The listing builds one solid part. Answer for the finished solid, in the listing's coordinates (mm). A direction names the side the tool comes from. Round coordinates to 2 decimals unless told otherwise and drop trailing zeros. Loops run counter-clockwise (first coordinate to the right, second up) from the corner with the lowest first, then second, coordinate; pieces in that order, holes last. Notation, with made-up numbers: (31.5, -9) - (49.5, -9) arc R8 ccw to (49.5, -1) - close; hole circle Ø10 at (-32.75, 68). An arc over 180 degrees is marked (long way). One line per item, written item: value.
Autodesk Inventor part; units mm, degrees
ref_plane "YZ Plane" through (0, 0, 0) normal (1, 0, 0) x (0, 1, 0)
ref_plane "XY Plane" through (0, 0, 0) normal (0, 0, 1) x (1, 0, 0)
sketch "Sketch1" plane through (0, 0, 0) normal (0, 1, 0) x (-1, 0, 0)
  circle A0 centre (0, 0) radius 10
  circle A1 centre (0, 0) radius 12.5
  line L0 (12.5, 0) -> (12.5, 50)
  line L1 (-12.5, 0) -> (-12.5, 50)
  line L2 (-12.5, 50) -> (12.5, 50)
  dimension "d0" = 20
  dimension "d1" = 25
  dimension "d2" = 50
extrude "Extrusion1" add sketch "Sketch1" along normal blind 15
sketch "Sketch3" plane through (-12.5, 0, 50) normal (0, 0, 1) x (1, 0, 0)
  point P0 (12.5, 0)
sketch "Sketch4" plane through (-12.5, 0, 50) normal (0, 0, 1) x (1, 0, 0)
  line L0 (25, 0) -> (25, 15)
  line L1 (25, 0) -> (25, 15)
  line L2 (0, 15) -> (25, 15)
  line L3 (25, 15) -> (0, 15)
  line L4 (0, 0) -> (0, 15)
  line L5 (0, 15) -> (0, 0)
  line L6 (0, 0) -> (25, 0)
  line L7 (0, 0) -> (25, 0)
  point P0 (12.5, 0)
extrude "Extrusion3" add sketch "Sketch4" along normal blind 25
sketch "Sketch9" plane through (0, 0, 0) normal (0, -1, 0) x (1, 0, 0)
  line L0 (-12.5, 25) -> (-22.5, 25)
  line L1 (-12.5, 25) -> (12.5, 25)
  line L2 (12.5, 0) -> (12.5, 75)
  line L3 (-12.5, 25) -> (-12.5, 75)
  line L4 (-12.5, 25) -> (-12.5, 75)
  line L5 (-12.5, 75) -> (12.5, 75)
  line L6 (-12.5, 75) -> (12.5, 75)
  line L7 (12.5, 75) -> (12.5, 25)
  line L8 (12.5, 0) -> (12.5, 30)
  line L9 (-12.5, 25) -> (-10.5, 25)
  line L10 (-10.5, 25) -> (-10.5, 75)
  line L11 (-12.5, 75) -> (-12.5, 25)
  line L12 (-10.5, 25) -> (12.5, 30)
  line L13 (-10.5, 25) -> (-10.5, 35)
  line L14 (-10.5, 35) -> (12.5, 35)
  point P0 (0, 0)
  point P1 (12.5, 35)
  dimension "d50" = 30
  dimension "d51" = 2
  dimension "d74" = 10
extrude "Extrusion7" add sketch "Sketch9" along normal blind 13 contours L10 L14 L2 L12
sketch "Sketch10" plane through (0, -13, 0) normal (0, -1, 0) x (1, 0, 0)
  point P0 (0, 0)
ref_plane "Work Plane1" through (0, 7.5, 0) normal (0, 1, 0) x (-1, 0, 0)
mirror "Mirror1" about plane through (0, 7.5, 0) normal (0, 1, 0) of "Extrusion7"
sketch "Sketch15" plane through (-10.5, 15, 25) normal (0.2124296, 0, -0.9771764) x (-0.9771764, 0, -0.2124296)
  line L0 (-23.5372, 0) -> (-23.5372, 13)
  line L1 (-14.7001, 13) -> (-18.6088, 13)
  line L2 (-23.5372, 0) -> (-18.5372, 0)
  line L3 (-18.5372, 0) -> (-18.5372, 13)
  line L4 (-18.5372, 13) -> (-23.5372, 13)
  line L5 (-23.5372, 13) -> (-23.5372, 0)
  line L6 (-23.5372, -28) -> (-24.5994, -28)
  line L7 (-18.6088, -28) -> (-18.6088, 13)
  line L8 (-23.5372, -28) -> (-18.6088, -28)
  line L9 (-18.6088, -28) -> (-18.6088, -15)
  line L10 (-18.6088, -15) -> (-23.5372, -15)
  line L11 (-23.5372, -15) -> (-23.5372, -28)
  point P0 (-4.9496, -15)
  point P1 (-33.0965, -28)
  point P2 (-18.6088, 0)
  point P3 (-23.5372, 13)
  dimension "d66" = 5
extrude "Extrusion9" add sketch "Sketch15" along normal blind 2 contours L0 L4 L7 L2 | L8 L11 L10 L7
sketch "Sketch16" plane through (0, 15, 0) normal (0, 1, 0) x (1, 0, 0)
  circle A0 centre (0, 0) radius 10
  circle A1 centre (0, 0) radius 12.5
  dimension "d69" = 25
extrude "Extrusion10" add sketch "Sketch16" along normal blind 2
sketch "Sketch17" plane through (0, 0, 0) normal (0, -1, 0) x (1, 0, 0)
  circle A0 centre (0, 0) radius 10
  circle A1 centre (0, 0) radius 10
  circle A2 centre (0, 0) radius 12.5
extrude "Extrusion11" add sketch "Sketch17" along normal blind 2
sketch "Sketch18" plane through (-12.5, 0, 0) normal (-1, 0, 0) x (0, 0, 1)
  point P0 (0, 0)
sketch "Sketch19" plane through (0, 0, 0) normal (0, -1, 0) x (1, 0, 0)
  line L0 (-12.5, 75) -> (12.5, 75)
  line L1 (12.5, 35) -> (-10.5, 35)
  line L2 (-12.5, 75) -> (12.5, 75)
  line L3 (12.5, 75) -> (12.5, 35)
  line L4 (12.5, 35) -> (-12.5, 35)
  line L5 (-12.5, 35) -> (-12.5, 75)
  point P0 (0, 0)
extrude "Extrusion12" add sketch "Sketch19" along normal blind 2.5
sketch "Sketch20" plane through (0, 15, 0) normal (0, 1, 0) x (1, 0, 0)
  line L0 (12.5, -75) -> (-12.5, -75)
  line L1 (12.5, -35) -> (12.5, -75)
  line L2 (-12.5, -75) -> (12.5, -75)
  line L3 (12.5, -75) -> (12.5, -35)
  line L4 (12.5, -35) -> (-12.5, -35)
  line L5 (-12.5, -35) -> (-12.5, -75)
  point P0 (0, 0)
extrude "Extrusion13" add sketch "Sketch20" along normal blind 2.5
sketch "Sketch21" plane through (-12.5, 0, 75) normal (0, 0, 1) x (1, 0, 0)
  line L0 (25, -2.5) -> (0, -2.5)
  line L1 (0, -2.5) -> (25, -2.5)
  line L2 (25, -2.5) -> (25, 17.5)
  line L3 (25, 17.5) -> (0, 17.5)
  line L4 (0, 17.5) -> (0, -2.5)
  point P0 (12.5, 0)
extrude "Extrusion14" add sketch "Sketch21" along normal blind 30
sketch "Sketch22" plane through (-12.5, 0, 0) normal (-1, 0, 0) x (0, 0, 1)
  line L0 (35, 15) -> (35, 17.5)
  line L1 (35, -2.5) -> (105, -2.5)
  line L2 (35, 17.5) -> (45, 17.5)
  line L3 (45, 17.5) -> (45, -2.5)
  line L4 (45, -2.5) -> (35, -2.5)
  line L5 (35, -2.5) -> (35, 17.5)
  line L6 (45, 7.5) -> (50, 7.5)
  line L7 (45, 5) -> (50, 5)
  line L8 (50, 5) -> (50, 10)
  line L9 (50, 10) -> (45, 10)
  line L10 (45, 10) -> (45, 5)
  line L11 (45, 5) -> (50, 10) construction
  line L12 (50, 5) -> (45, 10) construction
  line L13 (50, 7.5) -> (58, 7.5)
  line L14 (63, 5) -> (58, 5)
  line L15 (58, 5) -> (58, 10)
  line L16 (58, 10) -> (63, 10)
  line L17 (63, 10) -> (63, 5)
  line L18 (63, 5) -> (58, 10) construction
  line L19 (58, 5) -> (63, 10) construction
  line L20 (63, 7.5) -> (71, 7.5)
  line L21 (76, 5) -> (71, 5)
  line L22 (71, 5) -> (71, 10)
  line L23 (71, 10) -> (76, 10)
  line L24 (76, 10) -> (76, 5)
  line L25 (76, 5) -> (71, 10) construction
  line L26 (71, 5) -> (76, 10) construction
  line L27 (76, 7.5) -> (84, 7.5)
  line L28 (89, 5) -> (84, 5)
  line L29 (84, 5) -> (84, 10)
  line L30 (84, 10) -> (89, 10)
  line L31 (89, 10) -> (89, 5)
  line L32 (89, 5) -> (84, 10) construction
  line L33 (84, 5) -> (89, 10) construction
  line L34 (89, 7.5) -> (97, 7.5)
  line L35 (102, 5) -> (97, 5)
  line L36 (97, 5) -> (97, 10)
  line L37 (97, 10) -> (102, 10)
  line L38 (102, 10) -> (102, 5)
  line L39 (102, 5) -> (97, 10) construction
  line L40 (97, 5) -> (102, 10) construction
  point P0 (0, 0)
  point P1 (47.5, 7.5)
  point P2 (60.5, 7.5)
  point P3 (73.5, 7.5)
  point P4 (86.5, 7.5)
  point P5 (99.5, 7.5)
  dimension "d81" = 10
  dimension "d82" = 5
  dimension "d83" = 5
  dimension "d84" = 8
  dimension "d85" = 5
  dimension "d86" = 8
  dimension "d87" = 8
  dimension "d88" = 8
extrude "Extrusion15" cut sketch "Sketch22" against normal blind 30 contours L9 L8 L6 L3 | L3 L6 L8 L7 | L14 L15 L16 L17 | L21 L22 L23 L24 | L28 L29 L30 L31 | L35 L36 L37 L38
properties part number "Part10copycopy"
1) Consider L1, parallel to X at y = 6, z = 0; L2, parallel to Z at x = 0, y = -1.05; L3, parallel to Z at x = 10.25, y = 7. Determine where each line is inside the solid, lowest interval first.
Final values:
L1: -12.5 to -10, 10 to 12.5
L2: -12.5 to -10, 10 to 12.5, 27.28 to 105
L3: -7.15 to 45, 50 to 58, 63 to 71, 76 to 84, 89 to 97, 102 to 105
2) A cutting plane is placed at B-B on x = -1.75. Give the number of separate pieces and of enclosed holes in the cut face, and give its area (3 significant figures).
Final values:
separate pieces: 2
enclosed holes: 5
area: 1,920 mm2
3) Each of these flat-tipped pins is pushed along its axis until it touches: pin 1 Ø1.5 at (x, z) = (-5, 98.5) entering from -Y; pin 2 Ø12.5 at (x, z) = (-2, 52.5) entering from +Y; pin 3 Ø6 at (x, z) = (10, 17) entering from -Y. Where does it stop, or does it pass through?
Final values:
pin 1: y = -2.5
pin 2: y = 17.5
pin 3: y = 0
4) For a pull along Y with two mould halves and no side action, classify faces 5 (the flat face through (0, 8, 76)), 6 (the flat face through (1, -8, 35)), 7 (the flat face through (1, -13, 31)) as released by +Y, released by -Y, zero draft, split by the parting line, or undercut.
Final values:
face 5: undercut
face 6: zero draft
face 7: released by -Y
5) For faces 1 (the flat face through (0, 17.5, 70)), 2 (the flat face through (0, 10, 73)), 3 (the flat face through (-0.1, 17, -10.2)), 4 (the flat face through (-0.1, -2, 10.2)), determine the directions among +Z, -Z, +X, -X, +Y, -Y from which every point of the face is accessible in a straight line to the end or side of a thin tool.
Final values:
face 1: +Z, +X, -X, +Y
face 2: +X, -X
face 3: -Z, +X, -X, +Y
face 4: -Z, +X, -X, -Y
6) A cutting plane is placed at A-A on y = 23. Give the vertices of the cut face in (x, z).
Final values:
outline: (-10.5, 25) - (7.68, 28.95) - (8.11, 27) - (12.92, 28.05) - (12.5, 30) - (12.5, 35) - (-10.5, 35) - close
